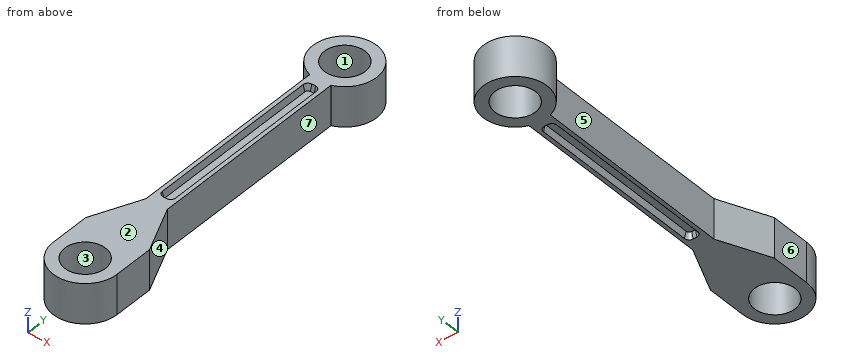
from build123d import *

# Parameters (mm, degrees)
BOSS_EXTRUDE5_DEPTH      = 6.35
BOSS_EXTRUDE5_DEPTH_BACK = 6.35
SKETCH2_R                = 6.477
CUT_EXTRUDE1_DEPTH       = 2.032
CUT_EXTRUDE1_DRAFT       = -15
MIRROR1_COPY_1_DEPTH     = 2.032
MIRROR1_COPY_1_DRAFT     = -15


with BuildPart() as part:
    # Sketch2 → Boss-Extrude5 (new, two sides: drawn at the far end of the back side and taken through both)
    with BuildSketch(Plane.XY.offset(-BOSS_EXTRUDE5_DEPTH_BACK)):
        with BuildLine():
            Line((10.16, -90.575195917), (10.16, -77.875195917))
            Line((10.16, -77.875195917), (3.394151371, -62.607190679))
            Line((3.394151371, -62.607190679), (3.394151371, 1.448513754))
            ThreePointArc((3.394151371, 1.448513754), (0, 21.184804083), (-3.394151371, 1.448513754))
            Line((-3.394151371, 1.448513754), (-3.394151371, -62.607190679))
            Line((-3.394151371, -62.607190679), (-10.16, -77.875195917))
            Line((-10.16, -77.875195917), (-10.16, -90.575195917))
            ThreePointArc((-10.16, -90.575195917), (0, -100.735195917), (10.16, -90.575195917))
        make_face()
        with Locations((0, 11.024804083)):
            Circle(SKETCH2_R, mode=Mode.SUBTRACT)
        with Locations((0, -90.575195917)):
            Circle(SKETCH2_R, mode=Mode.SUBTRACT)
    extrude(amount=BOSS_EXTRUDE5_DEPTH + BOSS_EXTRUDE5_DEPTH_BACK)


with BuildPart() as cut_extrude1_tool:
    # Sketch3 → Cut-Extrude1 (with draft: the straight prism first)
    with BuildSketch(Plane.XY.offset(6.35)):
        with BuildLine():
            ThreePointArc((2.124155322, -2.691195917), (1.677786057, -1.613565183), (0.600155322, -1.167195917))
            Line((0.600155322, -1.167195917), (-0.600155322, -1.167195917))
            ThreePointArc((-0.600155322, -1.167195917), (-1.677786057, -1.613565183), (-2.124155322, -2.691195917))
            Line((-2.124155322, -2.691195917), (-2.124155322, -57.809195917))
            ThreePointArc((-2.124155322, -57.809195917), (-1.677786057, -58.886826652), (-0.600155322, -59.333195917))
            Line((-0.600155322, -59.333195917), (0.600155322, -59.333195917))
            ThreePointArc((0.600155322, -59.333195917), (1.677786057, -58.886826652), (2.124155322, -57.809195917))
            Line((2.124155322, -57.809195917), (2.124155322, -2.691195917))
        make_face()
    extrude(amount=-CUT_EXTRUDE1_DEPTH)
    # Cut-Extrude1: the draft: its side faces are tilted about the plane it starts from
    cut_extrude1_sides = [cut_extrude1_tool.faces().sort_by_distance(p)[0] for p in [
        (2.124155322, -30.250195917, 5.334),
        (1.677786057, -1.613565183, 5.334),
        (0, -1.167195917, 5.334),
        (-1.677786057, -1.613565183, 5.334),
        (-2.124155322, -30.250195917, 5.334),
        (-1.677786057, -58.886826652, 5.334),
        (0, -59.333195917, 5.334),
        (1.677786057, -58.886826652, 5.334),
    ]]
    draft(cut_extrude1_sides, Plane.XY.offset(6.35), CUT_EXTRUDE1_DRAFT)


with BuildPart() as part_1:
    add(part.part)

    # Cut-Extrude1: cut by cut_extrude1_tool
    add(cut_extrude1_tool.part, mode=Mode.SUBTRACT)


with BuildPart() as mirror1_copy_1_tool:
    # Mirror1 copy 1 sketch → Mirror1 copy 1 (with draft: the straight prism first)
    with BuildSketch(Plane(origin=(0, 0, -6.35), x_dir=(1, 0, 0), z_dir=(0, 0, -1))):
        with BuildLine():
            ThreePointArc((2.124155322, 2.691195917), (1.677786057, 1.613565183), (0.600155322, 1.167195917))
            Line((0.600155322, 1.167195917), (-0.600155322, 1.167195917))
            ThreePointArc((-0.600155322, 1.167195917), (-1.677786057, 1.613565183), (-2.124155322, 2.691195917))
            Line((-2.124155322, 2.691195917), (-2.124155322, 57.809195917))
            ThreePointArc((-2.124155322, 57.809195917), (-1.677786057, 58.886826652), (-0.600155322, 59.333195917))
            Line((-0.600155322, 59.333195917), (0.600155322, 59.333195917))
            ThreePointArc((0.600155322, 59.333195917), (1.677786057, 58.886826652), (2.124155322, 57.809195917))
            Line((2.124155322, 57.809195917), (2.124155322, 2.691195917))
        make_face()
    extrude(amount=-MIRROR1_COPY_1_DEPTH)
    # Mirror1 copy 1: the draft: its side faces are tilted about the plane it starts from
    mirror1_copy_1_sides = [mirror1_copy_1_tool.faces().sort_by_distance(p)[0] for p in [
        (2.124155322, -30.250195917, -5.334),
        (1.677786057, -1.613565183, -5.334),
        (0, -1.167195917, -5.334),
        (-1.677786057, -1.613565183, -5.334),
        (-2.124155322, -30.250195917, -5.334),
        (-1.677786057, -58.886826652, -5.334),
        (0, -59.333195917, -5.334),
        (1.677786057, -58.886826652, -5.334),
    ]]
    draft(mirror1_copy_1_sides, Plane(origin=(0, 0, -6.35), x_dir=(1, 0, 0), z_dir=(0, 0, -1)), MIRROR1_COPY_1_DRAFT)


with BuildPart() as part_2:
    add(part_1.part)

    # Mirror1 copy 1: cut by mirror1_copy_1_tool
    add(mirror1_copy_1_tool.part, mode=Mode.SUBTRACT)


solid = part_2.part
Design review of the part built by this model. Coordinates are the model's own, in mm. Face numbers are marked on the shaded views. A direction names the side the tool comes from. Coordinates: 2 decimals unless noted, no trailing zeros. Order: outer loops, then holes, each group sorted by start corner. A loop starts at its lowest first (then second) coordinate and runs counter-clockwise, first axis right, second up. Notation, with made-up numbers: M -5,51 L 29,51 A27 cw 29,76 Z; hole C 0,61 d6. An arc over 180 degrees is marked long. Use a Markdown table: item, result.
(1) Add section A-A (x = -8.5). Give the boundary of the cut face in (y, z).
Worked answers:
| item | result |
|---|---|
| outline | M -96.14,-6.35 L -74.13,-6.35 L -74.13,6.35 L -96.14,6.35 Z; M 5.46,-6.35 L 16.59,-6.35 L 16.59,6.35 L 5.46,6.35 Z |
(2) Draft analysis for pull direction X (two halves, no side actions). For the marked faces 1, 2, 3 and 4, state which applies: released by +X, released by -X, zero draft, split by the parting line, or undercut.
Worked answers:
| item | result |
|---|---|
| face 1 | undercut |
| face 2 | zero draft |
| face 3 | undercut |
| face 4 | released by +X |
(3) Add section B-B (y = 6.5). Give the boundary of the cut face in (x, z), then the cut area to 3 significant figures.
Worked answers:
| item | result |
|---|---|
| outline | M -9.1,-6.35 L -4.63,-6.35 L -4.63,6.35 L -9.1,6.35 Z; M 4.63,-6.35 L 9.1,-6.35 L 9.1,6.35 L 4.63,6.35 Z |
| area | 113 mm2 |
(4) Wall thickness on probe 1 along Y at (x, z) = (0, -3.25); probe 2 along Y at (x, z) = (5.5, 3.5); probe 3 along Y at (x, z) = (4.5, -1.75): over which ranges is each line inside the solid? List them lowest first.
Worked answers:
| item | result |
|---|---|
| probe 1 | y = -100.74 to -97.05, -84.1 to 4.55, 17.5 to 21.18 |
| probe 2 | y = -99.12 to -94, -87.15 to -67.36, 2.48 to 7.6, 14.45 to 19.57 |
| probe 3 | y = -99.68 to -95.23, -85.92 to -65.1, 1.92 to 6.37, 15.68 to 20.13 |
(5) Add section D-D (y = -36.5). Give the boundary of the cut face in (x, z), then the cut area to 3 significant figures.
Worked answers:
| item | result |
|---|---|
| outline | M -3.39,-6.35 L -2.12,-6.35 L -1.58,-4.32 L 1.58,-4.32 L 2.12,-6.35 L 3.39,-6.35 L 3.39,6.35 L 2.12,6.35 L 1.58,4.32 L -1.58,4.32 L -2.12,6.35 L -3.39,6.35 Z |
| area | 71.2 mm2 |
(6) For P1, Ø4, axis at x = -3.5, z = -2, coming from the -Y side; P2, Ø1, axis at y = -33.5, z = -5, coming from the -X side; P3, Ø3.5, axis at x = -1, y = -27.5, coming from the -Z side; P4, Ø4, axis at y = -38.5, z = 1, coming from the +X side, all flat-tipped, find the tip position at first contact; note any pin that passes through.
Worked answers:
| item | result |
|---|---|
| P1 | stops at y = -100.62 |
| P2 | stops at x = -3.39 |
| P3 | stops at z = -6.35 |
| P4 | stops at x = 3.39 |
(7) Add section C-C (z = 1.75). Give the boundary of the cut face in (x, y), then the cut area to 3 significant figures.
Worked answers:
| item | result |
|---|---|
| outline | M -10.16,-90.58 A10.16 ccw 10.16,-90.58 L 10.16,-77.88 L 3.39,-62.61 L 3.39,1.45 A10.16 ccw long -3.39,1.45 L -3.39,-62.61 L -10.16,-77.88 Z; hole C 0,-90.58 d12.95; hole C 0,11.02 d12.95 |
| area | 1,120 mm2 |
(8) For the marked faces 5, 6 and 7, list the 3-axis set-ups (+Z, -Z, +X, -X, +Y, -Y) from which the entire face can be reached by the end or side of a thin tool; tool diameter is ignored.
Worked answers:
| item | result |
|---|---|
| face 5 | +Z, -Z, -X |
| face 6 | +Z, -Z, -X, +Y, -Y |
| face 7 | +Z, -Z, +X |
